Could you check a few things on this model? Use its own coordinates, in mm. Give positions to 0.01 mm unless a question says otherwise; leave off trailing zeros. Loops run counter-clockwise (first coordinate to the right, second up) from the corner with the lowest first, then second, coordinate; pieces in that order, holes last. Notation, with made-up numbers: M 42,-20.5 L 58,-20.5 A24 cw 58,12.5 Z; hole C 69,6.25 d7. An arc over 180 degrees is marked long. Return JSON: item names as keys, results as strings. Group by question number.
1. If we section it at B-B (x = -5.5): Write out the boundary of the cut face in (y, z).
2. Please list where these lines run through material, in increasing order: line 1 (Y direction, x = 8.5, z = -16.5); line 2 (Y direction, x = 10, z = 15); line 3 (X direction, y = 12, z = 31).
3. If we section it at C-C (y = 35.5): Write out the boundary of the cut face in (x, z), plus the area to 3 significant figures.
4. If we section it at A-A (z = -28): Write out the boundary of the cut face in (x, y), plus the area to 3 significant figures.
5. For pin 1 (5 mm diameter, centred on x = 10.5, z = 23.5, fed in from -Y); pin 2 (5 mm diameter, centred on y = 13.5, z = 23.5, fed in from -X); pin 3 (5 mm diameter, centred on y = 27.5, z = 15, fed in from -X), each with a flat end and sliding along its axis, tell me the tip position at first contact or that it passes through.
```python
from build123d import *

# Parameters (mm, degrees)
BOSS_EXTRUDE1_DEPTH = 38.1
BOSS_EXTRUDE2_DEPTH = 76.2


with BuildPart() as part:
    # Sketch1 → Boss-Extrude1 (new, symmetric)
    with BuildSketch(Plane.XY):
        Polygon((-16.002, 38.1), (16.002, 0), (12.827, 0), (-19.177, 38.1), align=None)
    extrude(amount=BOSS_EXTRUDE1_DEPTH, both=True)

    # Sketch2 → Boss-Extrude2 (add)
    with BuildSketch(Plane.XY.offset(38.1)):
        Polygon((12.827, 0), (14.140484991, -1.563672608), (16.002, 0), align=None)
        Polygon((-16.002, 38.1), (-17.315484991, 39.663672608), (-19.177, 38.1), align=None)
    extrude(amount=-BOSS_EXTRUDE2_DEPTH)


solid = part.part
```
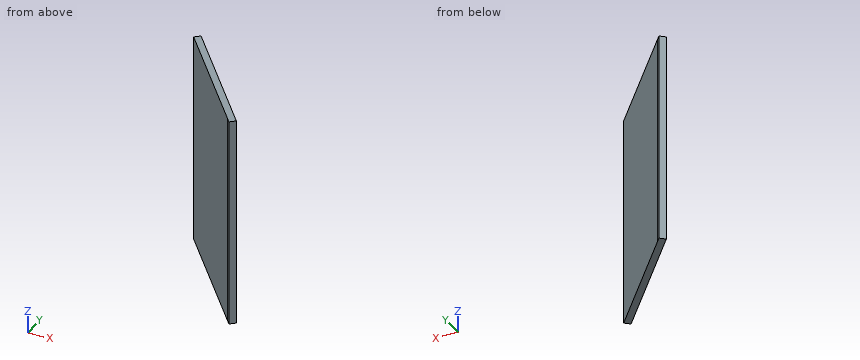
Answer:
{
 "1": {"outline": "M 21.82,-38.1 L 25.6,-38.1 L 25.6,38.1 L 21.82,38.1 Z"},
 "2": {"line 1": "y = 5.15 to 8.93", "line 2": "y = 3.37 to 7.15", "line 3": "x = 2.75 to 5.92"},
 "3": {"outline": "M -16.99,-38.1 L -13.82,-38.1 L -13.82,38.1 L -16.99,38.1 Z", "area": "242 mm²"},
 "4": {"outline": "M -19.18,38.1 L 14.14,-1.56 L 16,0 L -17.32,39.66 Z", "area": "126 mm²"},
 "5": {"pin 1": "stops at y = -0.21", "pin 2": "stops at x = -0.61", "pin 3": "stops at x = -12.37"}
}
